Design review of the part built by this model. Coordinates are the model's own, in mm. Give positions to 0.01 mm unless a question says otherwise; leave off trailing zeros. Loops run counter-clockwise (first coordinate to the right, second up) from the corner with the lowest first, then second, coordinate; pieces in that order, holes last. Notation, with made-up numbers: M 66.25,-19.5 L 96.25,-19.5 A20 cw 96.25,-10.5 Z; hole C 60,73.25 d9. An arc over 180 degrees is marked long. Answer as CSV lines item,"result".
```python
from build123d import *

# Parameters (mm, degrees)
BOSS_EXTRUDE1_DEPTH = 15
CHAMFER1_SIZE       = 2.5
SKETCH2_R           = 1.4
CUT_EXTRUDE1_DEPTH  = 40.667340007
SKETCH3_W           = 0.942684348
SKETCH3_H           = 15
CUT_EXTRUDE2_DEPTH  = 1


with BuildPart() as part:
    # Sketch1 → Boss-Extrude1 (new body)
    with BuildSketch(Plane.XY):
        with BuildLine():
            Line((-17.549928775, -4), (-32.549928775, -4))
            Line((-32.549928775, -4), (-32.549928775, -21))
            Line((-32.549928775, -21), (32.549928775, -21))
            Line((32.549928775, -21), (32.549928775, -4))
            Line((32.549928775, -4), (17.549928775, -4))
            ThreePointArc((17.549928775, -4), (0, -18), (-17.549928775, -4))
        make_face()
    extrude(amount=BOSS_EXTRUDE1_DEPTH)

    # Chamfer1
    chamfer1_edges = [part.edges().sort_by_distance(p)[0] for p in [
        (-32.549928775, -12.5, 15),
        (32.549928775, -12.5, 15),
        (-32.549928775, -12.5, 0),
        (32.549928775, -12.5, 0),
    ]]
    chamfer(chamfer1_edges, length=CHAMFER1_SIZE)

    # Sketch2 → Cut-Extrude1 (cut, through all)
    with BuildSketch(Plane(origin=(0, -4, 0), x_dir=(1, 0, 0), z_dir=(0, 1, 0))):
        with Locations(Location((27.488644481, -7.5, 0), (0, 0, 180))):
            Circle(SKETCH2_R)
        with Locations((-27.488644481, -7.5)):
            Circle(SKETCH2_R)
    extrude(amount=-CUT_EXTRUDE1_DEPTH, mode=Mode.SUBTRACT)

    # Sketch3 → Cut-Extrude2 (cut)
    with BuildSketch(Plane(origin=(0, -4, 0), x_dir=(1, 0, 0), z_dir=(0, 1, 0))):
        with Locations((-21.008394031, -7.5)):
            Rectangle(SKETCH3_W, SKETCH3_H)
    cut_extrude2 = extrude(amount=-CUT_EXTRUDE2_DEPTH, mode=Mode.SUBTRACT)

    # Mirror1: Cut-Extrude2 across plane
    add(cut_extrude2.mirror(Plane(origin=(0, 0, 0), x_dir=(0, 0, 1), z_dir=(1, 0, 0))), mode=Mode.SUBTRACT)


solid = part.part
```
1. We need section C-C, the plane z = 11. Write out the cut boundary in (x, y).
Answer block:
outline,"M -32.55,-21 L 32.55,-21 L 32.55,-4 L 21.48,-4 L 21.48,-5 L 20.54,-5 L 20.54,-4 L 17.55,-4 A18 cw -17.55,-4 L -20.54,-4 L -20.54,-5 L -21.48,-5 L -21.48,-4 L -32.55,-4 Z"
2. To check wall thickness, follow L1, parallel to X at y = -9.25, z = 9.75; L2, parallel to X at y = -13.5, z = 11.5; L3, parallel to Y at x = -10.5, z = 11. State the ranges of each line that lie inside material, in increasing order. Write a range as [from, to].
Answer block:
L1,"[-32.55, -15.44], [15.44, 32.55]"
L2,"[-32.55, -11.91], [11.91, 32.55]"
L3,"[-21, -14.62]"
3. We need section D-D, the plane y = -6.25. Write out the cut boundary in (x, z).
Answer block:
outline,"M -32.55,2.5 L -30.05,0 L -16.88,0 L -16.88,15 L -30.05,15 L -32.55,12.5 Z; M 16.88,0 L 30.05,0 L 32.55,2.5 L 32.55,12.5 L 30.05,15 L 16.88,15 Z; hole C -27.49,7.5 d2.8; hole C 27.49,7.5 d2.8"
4. We need section A-A, the plane y = -8.75. Write out the cut boundary in (x, z).
Answer block:
outline,"M -32.55,2.5 L -30.05,0 L -15.73,0 L -15.73,15 L -30.05,15 L -32.55,12.5 Z; M 15.73,0 L 30.05,0 L 32.55,2.5 L 32.55,12.5 L 30.05,15 L 15.73,15 Z; hole C -27.49,7.5 d2.8; hole C 27.49,7.5 d2.8"
5. We need section B-B, the plane z = 7.5. Write out the cut boundary in (x, y), plus the area to 3 significant figures.
Answer block:
outline,"M -32.55,-21 L -28.89,-21 L -28.89,-4 L -32.55,-4 Z; M -26.09,-21 L 26.09,-21 L 26.09,-4 L 21.48,-4 L 21.48,-5 L 20.54,-5 L 20.54,-4 L 17.55,-4 A18 cw -17.55,-4 L -20.54,-4 L -20.54,-5 L -21.48,-5 L -21.48,-4 L -26.09,-4 Z; M 28.89,-21 L 32.55,-21 L 32.55,-4 L 28.89,-4 Z"
area,"643 mm²"
6. The part is to be moulded in two halves that separate along X. For faces 1 (the cylindrical face through (0, -18, 7)), 2 (the flat face through (26, -4, 7)), 3 (the flat face through (-31.28, -12.38, 13.77)), say which applies: pulls with the +X half, pulls with the -X half, needs draft (parallel to the pull), parting line crosses it, or undercut.
Answer block:
face 1,"undercut"
face 2,"needs draft"
face 3,"pulls with the -X half"
7. For P1, Ø4, axis at x = 3, z = 8, coming from the +Y side; P2, Ø1.7, axis at x = 27.49, z = 7.5, coming from the +Y side, all flat-tipped, find the tip position at first contact; note any pin that passes through.
Answer block:
P1,"y = -17.29"
P2,"through"
